Autodesk Inventor part; units mm, degrees
ref_plane "YZ Plane" through (0, 0, 0) normal (1, 0, 0) x (0, 1, 0)
ref_plane "XZ Plane" through (0, 0, 0) normal (0, 1, 0) x (-1, 0, 0)
ref_plane "XY Plane" through (0, 0, 0) normal (0, 0, 1) x (1, 0, 0)
sketch "Náčrt1" plane through (0, 0, 0) normal (0, 1, 0) x (-1, 0, 0)
  line L0 (1.5, 0) -> (-9, 0)
  line L1 (0, -2.08) -> (0, 12.48)
  line L2 (-2.05, 10.3) -> (-2.05, 10)
  line L3 (-2.05, 10.3) -> (-2.15, 10.4)
  line L4 (-2.15, 10.4) -> (-5, 10.4)
  line L5 (-5, 10.4) -> (-5, 0)
  line L6 (-5, 0) -> (-3.46, 0)
  arc A0 (-3.5, 8.55) -> (-2.05, 10) centre (-3.5, 10) ccw
  line L7 (-3.46, 0) -> (-3.46, 7.0477)
  line L8 (-3.46, 7.0477) -> (-3.75, 7.55)
  line L9 (-3.75, 7.55) -> (-3.75, 8.55)
  line L10 (-3.5, 8.55) -> (-3.75, 8.55)
  line L11 (-5, 10.4) -> (-7.5, 10.4)
  line L12 (-7.5, 10.4) -> (-7.5, 8.9566)
  line L13 (-7.5, 8.9566) -> (-5, 10.4)
  line L14 (-5, 0) -> (-7.5, 0)
  line L15 (-7.5, 0) -> (-7.5, 1.4434)
  line L16 (-7.5, 1.4434) -> (-5, 0)
  line L17 (-3.46, 7.0477) -> (-3.46, 8.5506)
  point P0 (0, 0)
  dimension "d0" = 4.1
  dimension "d1" = 1.45
  dimension "d3" = 6.92
  dimension "d5" = 10
  dimension "d6" = 7.5
  dimension "d7" = 30
  dimension "d8" = 1
  dimension "d9" = 0.1
  dimension "d10" = 45
  dimension "d11" = 0.4
  dimension "d12" = 10.4
  dimension "d13" = 30
  dimension "d14" = 15
revolve "Rotace1" add sketch "Náčrt1" angle 360 about axis through (0, 0, -10) along (0, 0, 1) contours L0 L5 L4 L3 L2 A0 L10 L9 L8 L7 | L8 L9 L10 A0 L17
thread "Závit1"
sketch "Náčrt2" plane through (0, 0, 0) normal (0, 0, 1) x (1, 0, 0)
  circle A0 centre (0, 0) radius 5
  circle A1 centre (0, 0) radius 5
  line L0 (-5.7735, 0) -> (-2.8868, 5)
  line L1 (-2.8868, 5) -> (2.8868, 5)
  line L2 (2.8868, 5) -> (5.7735, 0)
  line L3 (5.7735, 0) -> (2.8868, -5)
  line L4 (2.8868, -5) -> (-2.8868, -5)
  line L5 (-2.8868, -5) -> (-5.7735, 0)
  dimension "d16" = 10
extrude "Vysunutí1" add sketch "Náčrt2" along normal blind 10.4 contours A0 L2 L3 | A0 L1 L2 | L3 L4 A0 | A0 L0 L1 | L4 L5 A0 | A0 L5 L0
revolve "Rotace2" cut sketch "Náčrt1" angle 360 about axis through (0, 0, -10) along (0, 0, 1) contours L0 L15 L16 | L13 L12 L11
revolve "Rotace3" cut sketch "Náčrt1" angle 360 about axis through (0, 0, -10) along (0, 0, 1) contours L8 L9 L10 A0 L17
chamfer "Zkosení1" distance 0.75 angle 45 1 edges at (-3.46, 0, 0)
equation "\"d17\" = d12"
Can you work these out from the model? Positions are in its coordinate system, mm. A direction names the side the tool comes from. Coordinates: 2 decimals unless noted, no trailing zeros. Write each loop counter-clockwise with the first axis right and the second up, starting at its lowest first coordinate (ties: lowest second). Pieces come first, ordered by that corner, then holes. Notation, with made-up numbers: (-20.5, -30.5) - (13.5, -30.5) arc R21 cw to (13.5, -8.5) - close; hole circle Ø9 at (4, 12). An arc over 180 degrees is marked (long way). Return JSON: item names as keys, results as strings. Group by question number.
Item 1: We'd pull the mould along X, two halves only. Please class faces 1 (the face through (3.3, 1.04, 3.94)), 2 (the face through (-2, -4, 0)), 3 (the face through (4.35, -2.465, 5.127)): pulls with the +X half, pulls with the -X half, needs draft (parallel to the pull), parting line crosses it, or undercut.
Item 2: If we section it at B-B (z = 7.25): Write out the boundary of the cut face in (x, y).
Item 3: Which directions (+Z, -Z, +X, -X, +Y, -Y) give clear straight access to the entire face, cutting with the end or side of a thin tool? Please do faces 4 (the face through (-3.746, 0.165, 8.057)), 5 (the face through (5.131, 0.113, 10.323)).
Item 4: I'm going to push flat-ended pins straight in: pin 1 Ø4.5 at (x, y) = (0, 0) entering from -Z; pin 2 Ø5 at (x, y) = (-4, 3) entering from -Z; pin 3 Ø2 at (y, z) = (2.5, 2) entering from +X. Where does each tip first touch, or does it pass through?
Item 5: Please list where these lines run through material, in increasing order: probe 1 along Y at (x, z) = (0, 8); probe 2 along Y at (x, z) = (0, 3.5); probe 3 along X at (y, z) = (-2.25, 6.25).
Item 6: If we section it at A-A (z = 4): Write out the boundary of the cut face in (x, y).
Return value:
{
 "1": {"face 1": "undercut", "face 2": "needs draft", "face 3": "pulls with the +X half"},
 "2": {"outline": "(-5.77, 0) - (-2.89, -5) - (2.89, -5) - (5.77, 0) - (2.89, 5) - (-2.89, 5) - close; hole circle Ø7.15 at (0, 0)"},
 "3": {"face 4": "none", "face 5": "+Z, +X"},
 "4": {"pin 1": "stops at z = 9.27", "pin 2": "stops at z = 0", "pin 3": "stops at x = 4.91"},
 "5": {"probe 1": "y = -5 to -3.75, 3.75 to 5", "probe 2": "y = -5 to -3.46, 3.46 to 5", "probe 3": "x = -4.47 to -2.63, 2.63 to 4.47"},
 "6": {"outline": "(-5.77, 0) - (-2.89, -5) - (2.89, -5) - (5.77, 0) - (2.89, 5) - (-2.89, 5) - close; hole circle Ø6.92 at (0, 0)"}
}
